Source: three-view drawing plus pictorial views. Frame: mm from the lowest corner of the part. Coordinates: 2 decimals unless noted, no trailing zeros. Loops run counter-clockwise (first coordinate to the right, second up) from the corner with the lowest first, then second, coordinate; pieces in that order, holes last. Notation, with made-up numbers: (-21.5, 37.5) -> (2.5, 37.5) arc R25 cw to (2.5, 75.5) -> close; hole circle Ø2 at (40, 10.25). An arc over 180 degrees is marked (long way). Answer as a JSON object with one key per item and string values. Group by question number.
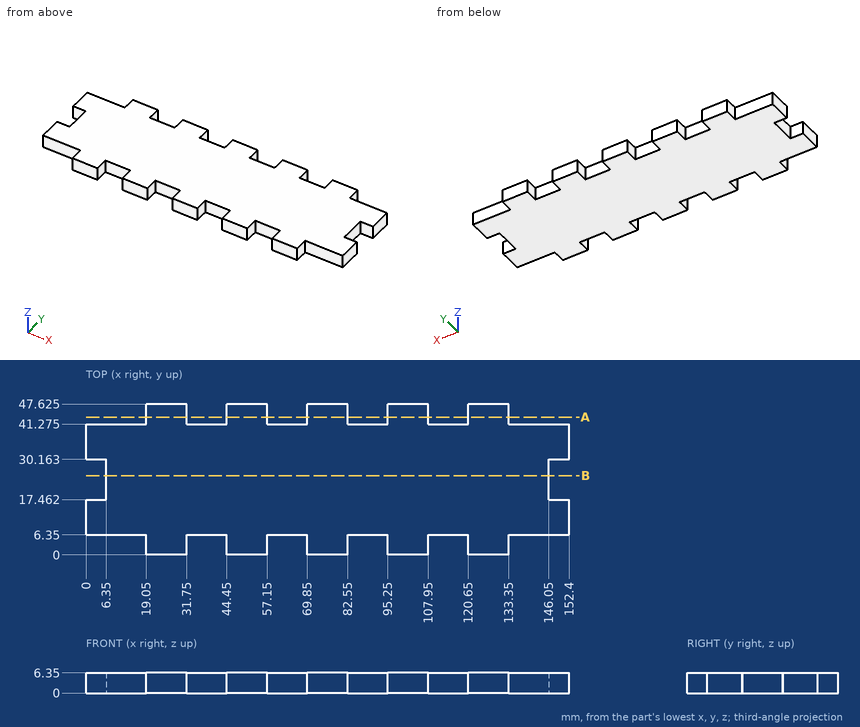
1. Section query A-A on y = 43.5. Return loops of the section in (x, z).
2. Ray query, L1, parallel to X at y = 41.5, z = 2; L2, parallel to X at y = 24.5, z = 3. Return the intervals inside material, ascending.
3. Pin query (flat end, axial travel): pin 1 Ø3 at (y, z) = (3.5, 3) entering from -X; pin 2 Ø1.9 at (x, z) = (36, 2) entering from -Y; pin 3 Ø1.9 at (y, z) = (24.5, 4) entering from +X. Return the tip coordinate at first contact, or that it passes through.
4. Section query B-B on y = 25. Return loops of the section in (x, z), then the cut area to 3 significant figures.
Solved:
{
 "1": {"outline": "(19.05, 0) -> (31.75, 0) -> (31.75, 6.35) -> (19.05, 6.35) -> close; (44.45, 0) -> (57.15, 0) -> (57.15, 6.35) -> (44.45, 6.35) -> close; (69.85, 0) -> (82.55, 0) -> (82.55, 6.35) -> (69.85, 6.35) -> close; (95.25, 0) -> (107.95, 0) -> (107.95, 6.35) -> (95.25, 6.35) -> close; (120.65, 0) -> (133.35, 0) -> (133.35, 6.35) -> (120.65, 6.35) -> close"},
 "2": {"L1": "19.05 to 31.75, 44.45 to 57.15, 69.85 to 82.55, 95.25 to 107.95, 120.65 to 133.35", "L2": "6.35 to 146.05"},
 "3": {"pin 1": "x = 19.05", "pin 2": "y = 6.35", "pin 3": "x = 146.05"},
 "4": {"outline": "(6.35, 0) -> (146.05, 0) -> (146.05, 6.35) -> (6.35, 6.35) -> close", "area": "887 mm^2"}
}
